Check sheet for the modelled part. Datum: model origin and axes. Units: mm. A direction names the side the tool comes from. Round coordinates to 2 decimals unless told otherwise and drop trailing zeros. Order: outer loops, then holes, each group sorted by start corner. A loop starts at its lowest first (then second) coordinate and runs counter-clockwise, first axis right, second up. Notation, with made-up numbers: (21.5, 22.25) -> (67.5, 22.25) arc R30 ccw to (67.5, 45.25) -> close; hole circle Ø7 at (67, 24). An arc over 180 degrees is marked (long way). Answer in a Markdown table with one row per item.
from build123d import *

# Parameters (mm, degrees)
SKETCH1_W           = 88
SKETCH1_H           = 125
BOSS_EXTRUDE1_DEPTH = 50
CUT_EXTRUDE1_DEPTH  = 117
FILLET1_R           = 3


with BuildPart() as part:
    # Sketch1 → Boss-Extrude1 (new body)
    with BuildSketch(Plane(origin=(0, 0, 0), x_dir=(1, 0, 0), z_dir=(0, 1, 0))):
        Rectangle(SKETCH1_W, SKETCH1_H)
    extrude(amount=BOSS_EXTRUDE1_DEPTH)

    # Sketch2 → Cut-Extrude1 (cut)
    with BuildSketch(Plane.XY.offset(58.5)):
        with BuildLine():
            Line((-41, 24.5), (-41, 66.5))
            Line((-41, 66.5), (41, 66.5))
            Line((41, 66.5), (41, 24.5))
            ThreePointArc((41, 24.5), (20.5, 4), (0, 24.5))
            ThreePointArc((0, 24.5), (-20.5, 4), (-41, 24.5))
        make_face()
    extrude(amount=-CUT_EXTRUDE1_DEPTH, mode=Mode.SUBTRACT)

    # Fillet1
    fillet1_edges = [part.edges().sort_by_distance(p)[0] for p in [
        (0, 24.5, 0),
    ]]
    fillet(fillet1_edges, radius=FILLET1_R)

    # Chamfer1
    # the kernel refuses this chamfer: 10 mm, written as the material it takes off along each edge
    with BuildSketch(Plane(origin=(-41, 50, 58.5), x_dir=(0, 0.027495876610586337, 0.9996219169112968), z_dir=(1, 0, 0)), Plane(origin=(-41, 50, -58.5), x_dir=(0, -0.9996219169112968, 0.027495876610586317), z_dir=(1, 0, 0))) as chamfer1_piece_1:
        with BuildLine():
            Line((10.286731952, 0), (-0.565471549, 10.271177935))
            Line((-0.565471549, 10.271177935), (-0.765395932, 10.26567876))
            ThreePointArc((-0.765395932, 10.26567876), (-0.341292271, 5.133978296), (-0.199924383, -0.005499175))
            Line((-0.199924383, -0.005499175), (0.005499175, -0.199924383))
            ThreePointArc((0.005499175, -0.199924383), (5.144976647, -0.058556496), (10.292231127, -0.199924383))
            Line((10.292231127, -0.199924383), (10.286731952, 0))
        make_face()
    extrude(amount=82, mode=Mode.SUBTRACT)
    with BuildSketch(Plane(origin=(41, 50, 58.5), x_dir=(0.9996219169112968, 0.027495876610586317, 0), z_dir=(0, 0, -1))) as chamfer1_piece_2:
        with BuildLine():
            Line((10.286731952, 0), (-0.565471549, 10.271177935))
            Line((-0.565471549, 10.271177935), (-0.765395932, 10.26567876))
            ThreePointArc((-0.765395932, 10.26567876), (-0.341292271, 5.133978296), (-0.199924383, -0.005499175))
            Line((-0.199924383, -0.005499175), (0.005499175, -0.199924383))
            ThreePointArc((0.005499175, -0.199924383), (5.144976647, -0.058556496), (10.292231127, -0.199924383))
            Line((10.292231127, -0.199924383), (10.286731952, 0))
        make_face()
    extrude(amount=117, mode=Mode.SUBTRACT)
    with BuildSketch(Plane(origin=(-41, 50, -58.5), x_dir=(0.027495876610586317, -0.9996219169112968, 0), z_dir=(0, 0, 1))) as chamfer1_piece_3:
        with BuildLine():
            Line((10.286731952, 0), (-0.565471549, -10.271177935))
            Line((-0.565471549, -10.271177935), (-0.765395932, -10.26567876))
            ThreePointArc((-0.765395932, -10.26567876), (-0.341292271, -5.133978296), (-0.199924383, 0.005499175))
            Line((-0.199924383, 0.005499175), (0.005499175, 0.199924383))
            ThreePointArc((0.005499175, 0.199924383), (5.144976647, 0.058556496), (10.292231127, 0.199924383))
            Line((10.292231127, 0.199924383), (10.286731952, 0))
        make_face()
    extrude(amount=117, mode=Mode.SUBTRACT)
    with BuildSketch(Plane(origin=(-41, 50, -58.5), x_dir=(0.027495876610586317, -0.9996219169112968, 0), z_dir=(0, 0, 1))) as chamfer1_piece_4a_section:
        with BuildLine():
            Line((10.286731952, 0), (-0.565471549, -10.271177935))
            Line((-0.565471549, -10.271177935), (-0.765395932, -10.26567876))
            ThreePointArc((-0.765395932, -10.26567876), (-0.341292271, -5.133978296), (-0.199924383, 0.005499175))
            Line((-0.199924383, 0.005499175), (0.005499175, 0.199924383))
            ThreePointArc((0.005499175, 0.199924383), (5.144976647, 0.058556496), (10.292231127, 0.199924383))
            Line((10.292231127, 0.199924383), (10.286731952, 0))
        make_face()
    chamfer1_piece_4a = extrude(amount=142.71682988, mode=Mode.PRIVATE)
    chamfer1_piece_4a = split(chamfer1_piece_4a, bisect_by=Plane(origin=(-44.297936268, 46.702063732, 58.5), z_dir=(0, 0, 1)), keep=Keep.TOP, mode=Mode.PRIVATE)
    with BuildSketch(Plane(origin=(-66.71682988, 50, 58.5), x_dir=(0, 0.027495876610586337, 0.9996219169112968), z_dir=(1, 0, 0))) as chamfer1_piece_4b_section:
        with BuildLine():
            Line((10.286731952, 0), (-0.565471549, 10.271177935))
            Line((-0.565471549, 10.271177935), (-0.765395932, 10.26567876))
            ThreePointArc((-0.765395932, 10.26567876), (-0.341292271, 5.133978296), (-0.199924383, -0.005499175))
            Line((-0.199924383, -0.005499175), (0.005499175, -0.199924383))
            ThreePointArc((0.005499175, -0.199924383), (5.144976647, -0.058556496), (10.292231127, -0.199924383))
            Line((10.292231127, -0.199924383), (10.286731952, 0))
        make_face()
    chamfer1_piece_4b = extrude(amount=107.71682988, mode=Mode.PRIVATE)
    chamfer1_piece_4b = split(chamfer1_piece_4b, bisect_by=Plane(origin=(-41, 46.702063732, 61.797936268), z_dir=(-1, 0, 0)), keep=Keep.TOP, mode=Mode.PRIVATE)
    chamfer1_piece_4 = chamfer1_piece_4a & chamfer1_piece_4b
    add(chamfer1_piece_4, mode=Mode.SUBTRACT)
    with BuildSketch(Plane(origin=(41, 50, 84.21682988), x_dir=(0.9996219169112968, 0.027495876610586317, 0), z_dir=(0, 0, -1))) as chamfer1_piece_5a_section:
        with BuildLine():
            Line((10.286731952, 0), (-0.565471549, 10.271177935))
            Line((-0.565471549, 10.271177935), (-0.765395932, 10.26567876))
            ThreePointArc((-0.765395932, 10.26567876), (-0.341292271, 5.133978296), (-0.199924383, -0.005499175))
            Line((-0.199924383, -0.005499175), (0.005499175, -0.199924383))
            ThreePointArc((0.005499175, -0.199924383), (5.144976647, -0.058556496), (10.292231127, -0.199924383))
            Line((10.292231127, -0.199924383), (10.286731952, 0))
        make_face()
    chamfer1_piece_5a = extrude(amount=142.71682988, mode=Mode.PRIVATE)
    chamfer1_piece_5a = split(chamfer1_piece_5a, bisect_by=Plane(origin=(44.297936268, 46.702063732, 58.5), z_dir=(0, 0, 1)), keep=Keep.TOP, mode=Mode.PRIVATE)
    with BuildSketch(Plane(origin=(-41, 50, 58.5), x_dir=(0, 0.027495876610586337, 0.9996219169112968), z_dir=(1, 0, 0))) as chamfer1_piece_5b_section:
        with BuildLine():
            Line((10.286731952, 0), (-0.565471549, 10.271177935))
            Line((-0.565471549, 10.271177935), (-0.765395932, 10.26567876))
            ThreePointArc((-0.765395932, 10.26567876), (-0.341292271, 5.133978296), (-0.199924383, -0.005499175))
            Line((-0.199924383, -0.005499175), (0.005499175, -0.199924383))
            ThreePointArc((0.005499175, -0.199924383), (5.144976647, -0.058556496), (10.292231127, -0.199924383))
            Line((10.292231127, -0.199924383), (10.286731952, 0))
        make_face()
    chamfer1_piece_5b = extrude(amount=107.71682988, mode=Mode.PRIVATE)
    chamfer1_piece_5b = split(chamfer1_piece_5b, bisect_by=Plane(origin=(41, 46.702063732, 61.797936268), z_dir=(1, 0, 0)), keep=Keep.TOP, mode=Mode.PRIVATE)
    chamfer1_piece_5 = chamfer1_piece_5a & chamfer1_piece_5b
    add(chamfer1_piece_5, mode=Mode.SUBTRACT)
    with BuildSketch(Plane(origin=(-41, 50, -58.5), x_dir=(0, -0.9996219169112968, 0.027495876610586317), z_dir=(1, 0, 0))) as chamfer1_piece_6a_section:
        with BuildLine():
            Line((10.286731952, 0), (-0.565471549, 10.271177935))
            Line((-0.565471549, 10.271177935), (-0.765395932, 10.26567876))
            ThreePointArc((-0.765395932, 10.26567876), (-0.341292271, 5.133978296), (-0.199924383, -0.005499175))
            Line((-0.199924383, -0.005499175), (0.005499175, -0.199924383))
            ThreePointArc((0.005499175, -0.199924383), (5.144976647, -0.058556496), (10.292231127, -0.199924383))
            Line((10.292231127, -0.199924383), (10.286731952, 0))
        make_face()
    chamfer1_piece_6a = extrude(amount=107.71682988, mode=Mode.PRIVATE)
    chamfer1_piece_6a = split(chamfer1_piece_6a, bisect_by=Plane(origin=(41, 46.702063732, -61.797936268), z_dir=(1, 0, 0)), keep=Keep.TOP, mode=Mode.PRIVATE)
    with BuildSketch(Plane(origin=(41, 50, 58.5), x_dir=(0.9996219169112968, 0.027495876610586317, 0), z_dir=(0, 0, -1))) as chamfer1_piece_6b_section:
        with BuildLine():
            Line((10.286731952, 0), (-0.565471549, 10.271177935))
            Line((-0.565471549, 10.271177935), (-0.765395932, 10.26567876))
            ThreePointArc((-0.765395932, 10.26567876), (-0.341292271, 5.133978296), (-0.199924383, -0.005499175))
            Line((-0.199924383, -0.005499175), (0.005499175, -0.199924383))
            ThreePointArc((0.005499175, -0.199924383), (5.144976647, -0.058556496), (10.292231127, -0.199924383))
            Line((10.292231127, -0.199924383), (10.286731952, 0))
        make_face()
    chamfer1_piece_6b = extrude(amount=142.71682988, mode=Mode.PRIVATE)
    chamfer1_piece_6b = split(chamfer1_piece_6b, bisect_by=Plane(origin=(44.297936268, 46.702063732, -58.5), z_dir=(0, 0, -1)), keep=Keep.TOP, mode=Mode.PRIVATE)
    chamfer1_piece_6 = chamfer1_piece_6a & chamfer1_piece_6b
    add(chamfer1_piece_6, mode=Mode.SUBTRACT)
    with BuildSketch(Plane(origin=(-66.71682988, 50, -58.5), x_dir=(0, -0.9996219169112968, 0.027495876610586317), z_dir=(1, 0, 0))) as chamfer1_piece_7a_section:
        with BuildLine():
            Line((10.286731952, 0), (-0.565471549, 10.271177935))
            Line((-0.565471549, 10.271177935), (-0.765395932, 10.26567876))
            ThreePointArc((-0.765395932, 10.26567876), (-0.341292271, 5.133978296), (-0.199924383, -0.005499175))
            Line((-0.199924383, -0.005499175), (0.005499175, -0.199924383))
            ThreePointArc((0.005499175, -0.199924383), (5.144976647, -0.058556496), (10.292231127, -0.199924383))
            Line((10.292231127, -0.199924383), (10.286731952, 0))
        make_face()
    chamfer1_piece_7a = extrude(amount=107.71682988, mode=Mode.PRIVATE)
    chamfer1_piece_7a = split(chamfer1_piece_7a, bisect_by=Plane(origin=(-41, 46.702063732, -61.797936268), z_dir=(-1, 0, 0)), keep=Keep.TOP, mode=Mode.PRIVATE)
    with BuildSketch(Plane(origin=(-41, 50, -84.21682988), x_dir=(0.027495876610586317, -0.9996219169112968, 0), z_dir=(0, 0, 1))) as chamfer1_piece_7b_section:
        with BuildLine():
            Line((10.286731952, 0), (-0.565471549, -10.271177935))
            Line((-0.565471549, -10.271177935), (-0.765395932, -10.26567876))
            ThreePointArc((-0.765395932, -10.26567876), (-0.341292271, -5.133978296), (-0.199924383, 0.005499175))
            Line((-0.199924383, 0.005499175), (0.005499175, 0.199924383))
            ThreePointArc((0.005499175, 0.199924383), (5.144976647, 0.058556496), (10.292231127, 0.199924383))
            Line((10.292231127, 0.199924383), (10.286731952, 0))
        make_face()
    chamfer1_piece_7b = extrude(amount=142.71682988, mode=Mode.PRIVATE)
    chamfer1_piece_7b = split(chamfer1_piece_7b, bisect_by=Plane(origin=(-44.297936268, 46.702063732, -58.5), z_dir=(0, 0, -1)), keep=Keep.TOP, mode=Mode.PRIVATE)
    chamfer1_piece_7 = chamfer1_piece_7a & chamfer1_piece_7b
    add(chamfer1_piece_7, mode=Mode.SUBTRACT)


solid = part.part
Item 1: Cross-section at C-C (y = 17.5). Record the boundary of the cut face in (x, z).
Result sheet:
| item | result |
|---|---|
| outline | (-44, -62.5) -> (44, -62.5) -> (44, 62.5) -> (-44, 62.5) -> close; hole (-39.77, -58.5) -> (39.77, -58.5) -> (39.77, 58.5) -> (-39.77, 58.5) -> close |
Item 2: Mould release check, pull along Z, two halves, no side actions. Record for faces 1 (the flat face through (-1, 0, -1)), 2 (the flat face through (-0.6, 42, -60.5)), 3 (the flat face through (-0.6, 42, 60.5)), 4 (the flat face through (-1, 22, -62.5)): pulls with the +Z half, pulls with the -Z half, needs draft (parallel to the pull), parting line crosses it, or undercut.
Result sheet:
| item | result |
|---|---|
| face 1 | needs draft |
| face 2 | undercut |
| face 3 | undercut |
| face 4 | pulls with the -Z half |
Item 3: Depth check by flat-ended pin: P1, Ø12, axis at x = 23, z = 14, coming from the +Y side. Enter the tip coordinate at first touch or a pass-through.
Result sheet:
| item | result |
|---|---|
| P1 | stops at y = 5.85 |
Item 4: Cross-section at B-B (x = 20.5). Record the boundary of the cut face in (y, z).
Result sheet:
| item | result |
|---|---|
| outline | (0, -62.5) -> (44, -62.5) -> (40, -58.5) -> (4, -58.5) -> (4, 58.5) -> (40, 58.5) -> (44, 62.5) -> (0, 62.5) -> close |
Item 5: Scan lines: line 1 (X direction, y = 15.5, z = -22); line 2 (X direction, y = 25, z = 17.5); line 3 (Z direction, x = 29.5, y = 20). Record each from-to range of solid material in increasing order. Write a range as [from, to].
Result sheet:
| item | result |
|---|---|
| line 1 | x = [-44, -38.92], [-1.67, 1.67], [38.92, 44] |
| line 2 | x = [-44, -41], [41, 44] |
| line 3 | z = [-62.5, -58.5], [58.5, 62.5] |
Item 6: Cross-section at D-D (x = -21). Record the boundary of the cut face in (y, z).
Result sheet:
| item | result |
|---|---|
| outline | (0, -62.5) -> (44, -62.5) -> (40, -58.5) -> (4.01, -58.5) -> (4.01, 58.5) -> (40, 58.5) -> (44, 62.5) -> (0, 62.5) -> close |
Item 7: Set-up check for faces 5 (the flat face through (-1, 22, 62.5)), 6 (the flat face through (1, 22, -58.5)): record each of +Z, -Z, +X, -X, +Y, -Y from which the full face is reachable in a straight line by a thin tool's end or side.
Result sheet:
| item | result |
|---|---|
| face 5 | +Z, +X, -X, +Y, -Y |
| face 6 | +Y |
Item 8: Cross-section at A-A (y = 30). Record the boundary of the cut face in (x, z).
Result sheet:
| item | result |
|---|---|
| outline | (-44, -62.5) -> (44, -62.5) -> (44, 62.5) -> (-44, 62.5) -> close; hole (-41, -58.5) -> (41, -58.5) -> (41, 58.5) -> (-41, 58.5) -> close |
